```python
from build123d import *

# Parameters (mm, degrees)
F0_W     = 129.54
F0_H     = 134.62
F0_W_2   = 120.904
F0_H_2   = 124.714
F1_DEPTH = 12.7
F2_R     = 3.175
F4_W     = 11.43
F4_H     = 2.159
F5_DEPTH = 1.016
F3_W     = 11.43
F3_H     = 2.159
F6_DEPTH = 1.016
F7_R     = 1.27
F8_R     = 0.508
F10_R    = 1.27


with BuildPart() as f1:
    # F0 (on Top) → F1 (new body)
    with BuildSketch(Plane.XY):
        Rectangle(F0_W, F0_H)
        Rectangle(F0_W_2, F0_H_2, mode=Mode.SUBTRACT)
    extrude(amount=F1_DEPTH)

    # F2
    f2_edges = [f1.edges().sort_by_distance(p)[0] for p in [
        (-60.452, 62.357, 6.35),
        (-60.452, -62.357, 6.35),
        (60.452, 62.357, 6.35),
        (60.452, -62.357, 6.35),
        (-64.77, 67.31, 6.35),
        (64.77, 67.31, 6.35),
        (-64.77, -67.31, 6.35),
        (64.77, -67.31, 6.35),
    ]]
    fillet(f2_edges, radius=F2_R)

    # F4 (on face) → F5 (join)
    with BuildSketch(Plane(origin=(60.452, 0, 0), x_dir=(0, -1, 0), z_dir=(-1, 0, 0))):
        with Locations((0.127, 11.6205)):
            Rectangle(F4_W, F4_H)
    extrude(amount=F5_DEPTH)

    # F3 (on face) → F6 (join)
    with BuildSketch(Plane.YZ.offset(-60.452)):
        with Locations((0.127, 11.6205)):
            Rectangle(F3_W, F3_H)
    extrude(amount=F6_DEPTH)

    # F7
    f7_edges = [f1.edges().sort_by_distance(p)[0] for p in [
        (0, -62.357, 12.7),
        (0, 62.357, 0),
        (-64.77, 0, 0),
        (-60.452, 32.512, 12.7),
    ]]
    fillet(f7_edges, radius=F7_R)

    # F8
    f8_edges = [f1.edges().sort_by_distance(p)[0] for p in [
        (-59.436, 5.842, 11.6205),
        (-59.436, -5.588, 11.6205),
        (-59.436, 0.127, 10.541),
        (-59.436, 0.127, 12.7),
        (59.436, 5.588, 11.6205),
        (59.436, -5.842, 11.6205),
        (59.436, -0.127, 12.7),
        (59.436, -0.127, 10.541),
    ]]
    fillet(f8_edges, radius=F8_R)

    # F10
    f10_edges = [f1.edges().sort_by_distance(p)[0] for p in [
        (0, 67.31, 12.7),
        (-63.840064, 66.380064, 12.7),
        (-64.77, 0, 12.7),
        (-63.840064, -66.380064, 12.7),
        (0, -67.31, 12.7),
        (63.840064, -66.380064, 12.7),
        (64.77, 0, 12.7),
        (63.840064, 66.380064, 12.7),
    ]]
    fillet(f10_edges, radius=F10_R)


solid = f1.part
```
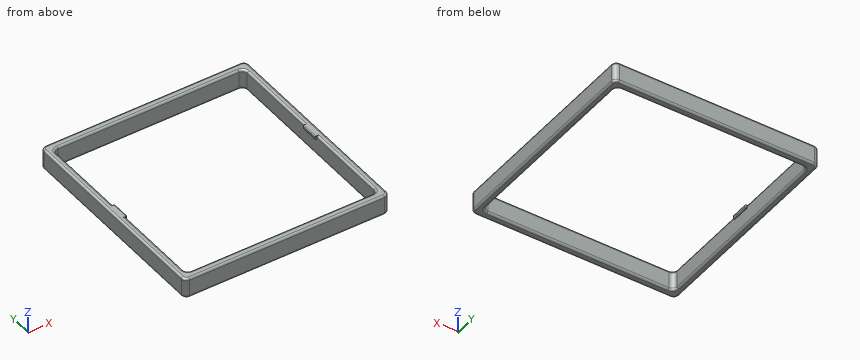
Input: part model. Units: mm. Frame: model coordinates. Round coordinates to 2 decimals unless told otherwise and drop trailing zeros. Loops run counter-clockwise (first coordinate to the right, second up) from the corner with the lowest first, then second, coordinate; pieces in that order, holes last. Notation, with made-up numbers: M -40,75.5 L -15,75.5 A35 ccw -15,111.5 Z; hole C -13.5,-35 d6. An arc over 180 degrees is marked long. Answer in a Markdown table with one row per item. Add a question column.
1. Ray query, probe 1 along Y at (x, z) = (-38, 7.5); probe 2 along X at (y, z) = (11.5, 7.5); probe 3 along Y at (x, z) = (57.5, 4.5). Return the intervals inside material, ascending.
2. Section B-B (y = 26). Output: boundary loops of the cut face in (x, z), and give its area (3 significant figures).
3. Contact query for flat-ended pins moving along their axis: pin 1 (0.5 mm diameter, centred on x = 60.5, z = 12, fed in from -Y); pin 2 (0.5 mm diameter, centred on x = -61, z = 12, fed in from +Y); pin 3 (12 mm diameter, centred on x = 51, y = 45, fed in from +Z). Output: stop coordinate, or through.
4. Section C-C (z = 5). Output: boundary loops of the cut face in (x, y) (3 decimals).
5. Section A-A (x = 47). Output: boundary loops of the cut face in (y, z).
Values follow:
| question | item | result |
|---|---|---|
| 1 | probe 1 | -67.31 to -62.36, 62.36 to 67.31 |
| 1 | probe 2 | -64.77 to -60.45, 60.45 to 64.77 |
| 1 | probe 3 | -67.31 to -62.35, 62.35 to 67.31 |
| 2 | outline | M -64.77,1.27 A1.27 ccw -63.5,0 L -61.72,0 A1.27 ccw -60.45,1.27 L -60.45,11.43 A1.27 ccw -61.72,12.7 L -63.5,12.7 A1.27 ccw -64.77,11.43 Z; M 60.45,1.27 A1.27 ccw 61.72,0 L 63.5,0 A1.27 ccw 64.77,1.27 L 64.77,11.43 A1.27 ccw 63.5,12.7 L 61.72,12.7 A1.27 ccw 60.45,11.43 Z |
| 2 | area | 107 mm^2 |
| 3 | pin 1 | y = -67.27 |
| 3 | pin 2 | y = 67.27 |
| 3 | pin 3 | through |
| 4 | outline | M -64.77,-64.135 A3.175 ccw -61.595,-67.31 L 61.595,-67.31 A3.175 ccw 64.77,-64.135 L 64.77,64.135 A3.175 ccw 61.595,67.31 L -61.595,67.31 A3.175 ccw -64.77,64.135 Z; hole M -60.452,-59.182 A3.175 ccw -57.277,-62.357 L 57.277,-62.357 A3.175 ccw 60.452,-59.182 L 60.452,59.182 A3.175 ccw 57.277,62.357 L -57.277,62.357 A3.175 ccw -60.452,59.182 Z |
| 5 | outline | M -67.31,1.27 A1.27 ccw -66.04,0 L -63.63,0 A1.27 ccw -62.36,1.27 L -62.36,11.43 A1.27 ccw -63.63,12.7 L -66.04,12.7 A1.27 ccw -67.31,11.43 Z; M 62.36,1.27 A1.27 ccw 63.63,0 L 66.04,0 A1.27 ccw 67.31,1.27 L 67.31,11.43 A1.27 ccw 66.04,12.7 L 63.63,12.7 A1.27 ccw 62.36,11.43 Z |
